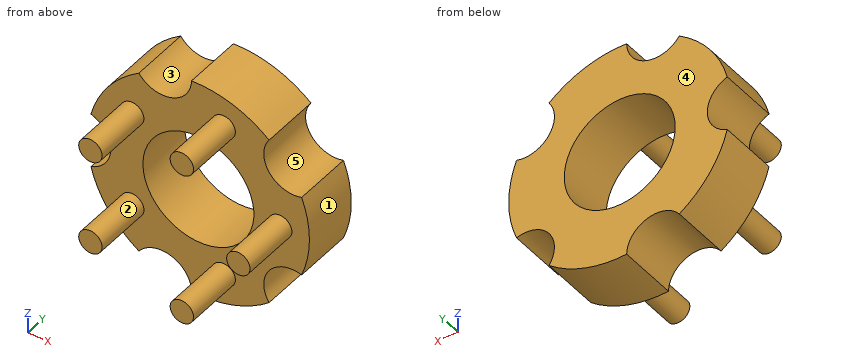
Autodesk Inventor part; units mm, degrees
ref_plane "YZ Plane" through (0, 0, 0) normal (1, 0, 0) x (0, 1, 0)
ref_plane "XZ Plane" through (0, 0, 0) normal (0, 1, 0) x (-1, 0, 0)
ref_plane "XY Plane" through (0, 0, 0) normal (0, 0, 1) x (1, 0, 0)
sketch "Эскиз1" plane through (0, 0, 0) normal (0, 1, 0) x (-1, 0, 0)
  circle A0 centre (0, 0) radius 9.5
  circle A1 centre (0, 0) radius 30
  circle A2 centre (0, 0) radius 20 construction
  circle A3 centre (19.9999, 0) radius 5
  circle A4 centre (6.1803, 19.021) radius 5
  circle A5 centre (-16.1803, 11.7557) radius 5
  circle A6 centre (-16.1803, -11.7557) radius 5
  circle A7 centre (6.1803, -19.021) radius 5
  dimension "d0" = 19
  dimension "d1" = 60
  dimension "d2" = 40
  dimension "d3" = 10
  dimension "d6" = 360
extrude "Выдавливание1" add sketch "Эскиз1" along normal blind 10
sketch "Эскиз2" plane through (0, 10, 0) normal (0, 1, 0) x (1, 0, 0)
  circle A0 centre (-6.1803, 19.021) radius 5
  circle A1 centre (16.1803, 11.7557) radius 5
  circle A2 centre (16.1803, -11.7557) radius 5
  circle A3 centre (-6.1803, -19.021) radius 5
  circle A4 centre (-19.9999, 0) radius 5
  circle A5 centre (0, 0) radius 30
  circle A6 centre (0, 0) radius 19
  dimension "d15" = 38
extrude "Выдавливание2" cut sketch "Эскиз2" against normal blind 10
sketch "Эскиз3" plane through (0, 10, 0) normal (0, 1, 0) x (1, 0, 0)
  circle A0 centre (0, 0) radius 9.5
  circle A1 centre (14, 0) radius 2
  circle A2 centre (4.3262, 13.3148) radius 2
  circle A3 centre (-11.3262, 8.229) radius 2
  circle A4 centre (-11.3262, -8.229) radius 2
  circle A5 centre (4.3262, -13.3148) radius 2
  dimension "d17" = 4
  dimension "d18" = 14
  dimension "d21" = 360
extrude "Выдавливание3" add sketch "Эскиз3" against normal blind 20 contours A1 | A2 | A3 | A4 | A5
properties part number "Ротор цевков"
Can you work these out from the model? Positions are in its coordinate system, mm. Face numbers are marked on the shaded views. A direction names the side the tool comes from. Round coordinates to 2 decimals unless told otherwise and drop trailing zeros. Loops run counter-clockwise (first coordinate to the right, second up) from the corner with the lowest first, then second, coordinate; pieces in that order, holes last. Notation, with made-up numbers: M -27.75,38.5 L -1.75,38.5 A17 cw -1.75,54.5 Z; hole C -2.5,-3 d7. An arc over 180 degrees is marked long. Answer as a JSON object with one key per item and string values. Group by question number.
Q1. Imagine slicing it at A-A, the plane z = 0. Please give me the cut outline in (x, y).
Q2. Imagine slicing it at B-B, the plane y = 7.5. Please give me the cut outline in (x, z), then the cut area to 3 significant figures.
Q3. On a 3-axis mill with a long thin cutter (end or side, diameter ignored), from which of +Z, -Z, +X, -X, +Y, -Y can I reach the whole of each face in a straight line? I mean the marked faces 1 and 2. Say none if no direction works.
Q4. Imagine slicing it at D-D, the plane y = -6.75. Please give me the cut outline in (x, z).
Q5. Imagine slicing it at C-C, the plane x = 0. Please give me the cut outline in (y, z), then the cut area to 3 significant figures.
Q6. Will these pins go through, and if not, where does the flat tip stop? pin 1 (5 mm diameter, centred on y = -4.5, z = 0.5, fed in from -X); pin 2 (4 mm diameter, centred on x = 11.5, z = -7, fed in from -Y); pin 3 (4 mm diameter, centred on x = 12, y = 1.5, fed in from +Z).
Q7. We'd pull the mould along Z, two halves only. Please class the marked faces 3, 4 and 5: +Z half, -Z half, draft (parallel to the pull), parting line (faces both ways), or undercut.
Q8. Please list where these lines run through material, in increasing order: L1, parallel to Z at x = 0, y = 5.75; L2, parallel to Y at x = -16, z = 8; L3, parallel to X at y = 6, z = 15.
Findings:
{
 "1": {"outline": "M -15,0 L -9.5,0 L -9.5,10 L -15,10 Z; M 9.5,0 L 12,0 L 12,-10 L 16,-10 L 16,0 L 19,0 L 19,10 L 9.5,10 Z"},
 "2": {"outline": "M -18.4,-4.74 A19 ccw -10.19,-16.04 A5 cw -1.18,-18.96 A19 ccw 12.1,-14.65 A5 cw 17.67,-6.98 A19 ccw 17.67,6.98 A5 cw 12.1,14.65 A19 ccw -1.18,18.96 A5 cw -10.19,16.04 A19 ccw -18.4,4.74 A5 cw Z; hole C 0,0 d19", "area": "714 mm2"},
 "3": {"face 1": "+X, +Y, -Y", "face 2": "-Y"},
 "4": {"outline": "C -11.33,-8.23 d4; C -11.33,8.23 d4; C 4.33,-13.31 d4; C 4.33,13.31 d4; C 14,0 d4"},
 "5": {"outline": "M 0,-19 L 10,-19 L 10,-9.5 L 0,-9.5 Z; M 0,9.5 L 10,9.5 L 10,19 L 0,19 Z", "area": "190 mm2"},
 "6": {"pin 1": "stops at x = 12", "pin 2": "stops at y = 0", "pin 3": "stops at z = 16.16"},
 "7": {"face 3": "+Z half", "face 4": "draft", "face 5": "undercut"},
 "8": {"L1": "z = -19 to -9.5, 9.5 to 19", "L2": "y = 0 to 10", "L3": "x = -11.66 to -9.15, -3.21 to 11.66"}
}
